from build123d import *

# Parameters (mm, degrees)
SKETCH_1_W                 = 310
SKETCH_1_H                 = 220
EXTRUDE_1_DEPTH            = 12
SKETCH_8_W                 = 310
SKETCH_8_H                 = 10
EXTRUDE_12_DEPTH           = 4
SKETCH_10_R                = 4
CUT_EXTRUDE_5_DEPTH        = 305
SKETCH_11_W                = 4
SKETCH_11_H                = 4
EXTRUDE_13_DEPTH           = 5
EXTRUDE_START              = 300
SKETCH_12_R                = 4
SKETCH_12_R_2              = 3
EXTRUDE_1_2_DEPTH          = 300
SPLIT_START                = -49.339622642
SPLIT_BODIES_2_OUTLINE_R   = 3
SPLIT_BODIES_2_DEPTH       = 100
SPLIT_START_2              = -149.339622642
SPLIT_BODIES_2_2_OUTLINE_R = 3
SPLIT_BODIES_2_2_DEPTH     = 50
SPLIT_START_3              = 100.660377358
SPLIT_BODIES_2_3_OUTLINE_R = 3
SPLIT_BODIES_2_3_DEPTH     = 50
SKETCH_14_W                = 50
SKETCH_14_H                = 8
SKETCH_14_W_2              = 100
EXTRUDE_14_DEPTH           = 12
SKETCH_15_W                = 5
SKETCH_15_H                = 220
EXTRUDE_15_DEPTH           = 5


# Read off the part's stored shape, not the designer's step: 分割2
with BuildPart() as part:
    # 草图1 → Extrude 1 (new body)
    with BuildSketch(Plane(origin=(0, 0, 0), x_dir=(1, 0, 0), z_dir=(0, 1, 0))):
        with Locations((0.660377358, 22.830188679)):
            Rectangle(SKETCH_1_W, SKETCH_1_H)
    extrude(amount=EXTRUDE_1_DEPTH)

    # 草图8 → 凸台-拉伸12 (add)
    with BuildSketch(Plane(origin=(0, 12, 0), x_dir=(1, 0, 0), z_dir=(0, 1, 0))):
        with Locations((0.660377358, 127.830188679)):
            Rectangle(SKETCH_8_W, SKETCH_8_H)
        with Locations((0.660377358, -82.169811321)):
            Rectangle(SKETCH_8_W, SKETCH_8_H)
    extrude(amount=EXTRUDE_12_DEPTH)

    # 草图10 → 切除-拉伸5 (cut)
    with BuildSketch(Plane(origin=(155.660377358, 0, 0), x_dir=(0, 0, -1), z_dir=(1, 0, 0))):
        with Locations((-77.169811321, 16)):
            Circle(SKETCH_10_R)
        with Locations((122.830188679, 16)):
            Circle(SKETCH_10_R)
    extrude(amount=-CUT_EXTRUDE_5_DEPTH, mode=Mode.SUBTRACT)

    # 草图11 → 凸台-拉伸13 (add)
    with BuildSketch(Plane(origin=(155.660377358, 0, 0), x_dir=(0, 0, -1), z_dir=(1, 0, 0))):
        with Locations((-79.169811321, 14)):
            Rectangle(SKETCH_11_W, SKETCH_11_H)
        with Locations((124.830188679, 14)):
            Rectangle(SKETCH_11_W, SKETCH_11_H)
    extrude(amount=-EXTRUDE_13_DEPTH)

    # 草图12 → Extrude 1 2 (add)
    # profile 1 of 2: a face of its own
    with BuildSketch(Plane(origin=(-149.339622642, 0, 0), x_dir=(0, 0, -1), z_dir=(1, 0, 0)).offset(EXTRUDE_START)):
        with Locations((-77.169811321, 16)):
            Circle(SKETCH_12_R)
        with Locations((-77.169811321, 16)):
            Circle(SKETCH_12_R_2, mode=Mode.SUBTRACT)
    # profile 2 of 2: a face of its own
    with BuildSketch(Plane(origin=(-149.339622642, 0, 0), x_dir=(0, 0, -1), z_dir=(1, 0, 0)).offset(EXTRUDE_START)):
        with Locations((122.830188679, 16)):
            Circle(SKETCH_12_R)
        with Locations((122.830188679, 16)):
            Circle(SKETCH_12_R_2, mode=Mode.SUBTRACT)
    extrude(amount=-EXTRUDE_1_2_DEPTH)

    # Split Bodies 2 outline → Split Bodies 2 (cut)
    # profile 1 of 2: a face of its own
    with BuildSketch(Plane.YZ.offset(SPLIT_START)):
        with BuildLine():
            Line((12, -122.830188679), (12, -118.830188679))
            Line((12, -118.830188679), (0, -118.830188679))
            Line((0, -118.830188679), (0, -126.830188679))
            Line((0, -126.830188679), (16, -126.830188679))
            ThreePointArc((16, -126.830188679), (18.828427125, -120.001761554), (12, -122.830188679))
        make_face()
        with Locations((16, -122.830188679)):
            Circle(SPLIT_BODIES_2_OUTLINE_R, mode=Mode.SUBTRACT)
    # profile 2 of 2: a face of its own
    with BuildSketch(Plane.YZ.offset(SPLIT_START)):
        with BuildLine():
            Line((0, 73.169811321), (12, 73.169811321))
            Line((12, 73.169811321), (12, 77.169811321))
            ThreePointArc((12, 77.169811321), (18.828427125, 74.341384196), (16, 81.169811321))
            Line((16, 81.169811321), (0, 81.169811321))
            Line((0, 81.169811321), (0, 73.169811321))
        make_face()
        with Locations((16, 77.169811321)):
            Circle(SPLIT_BODIES_2_OUTLINE_R, mode=Mode.SUBTRACT)
    extrude(amount=SPLIT_BODIES_2_DEPTH, mode=Mode.SUBTRACT)

    # Split Bodies 2 2 outline → Split Bodies 2 2 (cut)
    # profile 1 of 2: a face of its own
    with BuildSketch(Plane.YZ.offset(SPLIT_START_2)):
        with BuildLine():
            Line((12, -122.830188679), (12, -118.830188679))
            Line((12, -118.830188679), (0, -118.830188679))
            Line((0, -118.830188679), (0, -126.830188679))
            Line((0, -126.830188679), (16, -126.830188679))
            ThreePointArc((16, -126.830188679), (18.828427125, -120.001761554), (12, -122.830188679))
        make_face()
        with Locations((16, -122.830188679)):
            Circle(SPLIT_BODIES_2_2_OUTLINE_R, mode=Mode.SUBTRACT)
    # profile 2 of 2: a face of its own
    with BuildSketch(Plane.YZ.offset(SPLIT_START_2)):
        with BuildLine():
            Line((0, 73.169811321), (12, 73.169811321))
            Line((12, 73.169811321), (12, 77.169811321))
            ThreePointArc((12, 77.169811321), (18.828427125, 74.341384196), (16, 81.169811321))
            Line((16, 81.169811321), (0, 81.169811321))
            Line((0, 81.169811321), (0, 73.169811321))
        make_face()
        with Locations((16, 77.169811321)):
            Circle(SPLIT_BODIES_2_2_OUTLINE_R, mode=Mode.SUBTRACT)
    extrude(amount=SPLIT_BODIES_2_2_DEPTH, mode=Mode.SUBTRACT)

    # Split Bodies 2 3 outline → Split Bodies 2 3 (cut)
    # profile 1 of 2: a face of its own
    with BuildSketch(Plane.YZ.offset(SPLIT_START_3)):
        with BuildLine():
            Line((12, -122.830188679), (12, -118.830188679))
            Line((12, -118.830188679), (0, -118.830188679))
            Line((0, -118.830188679), (0, -126.830188679))
            Line((0, -126.830188679), (16, -126.830188679))
            ThreePointArc((16, -126.830188679), (18.828427125, -120.001761554), (12, -122.830188679))
        make_face()
        with Locations((16, -122.830188679)):
            Circle(SPLIT_BODIES_2_3_OUTLINE_R, mode=Mode.SUBTRACT)
    # profile 2 of 2: a face of its own
    with BuildSketch(Plane.YZ.offset(SPLIT_START_3)):
        with BuildLine():
            Line((0, 73.169811321), (12, 73.169811321))
            Line((12, 73.169811321), (12, 77.169811321))
            ThreePointArc((12, 77.169811321), (18.828427125, 74.341384196), (16, 81.169811321))
            Line((16, 81.169811321), (0, 81.169811321))
            Line((0, 81.169811321), (0, 73.169811321))
        make_face()
        with Locations((16, 77.169811321)):
            Circle(SPLIT_BODIES_2_3_OUTLINE_R, mode=Mode.SUBTRACT)
    extrude(amount=SPLIT_BODIES_2_3_DEPTH, mode=Mode.SUBTRACT)

    # 草图14 → 凸台-拉伸14 (add)
    with BuildSketch(Plane(origin=(0, 12, 0), x_dir=(1, 0, 0), z_dir=(0, 1, 0))):
        with Locations((-124.339622642, 122.830188679)):
            Rectangle(SKETCH_14_W, SKETCH_14_H)
        with Locations((125.660377358, 122.830188679)):
            Rectangle(SKETCH_14_W, SKETCH_14_H)
        with Locations((-124.339622642, -77.169811321)):
            Rectangle(SKETCH_14_W, SKETCH_14_H)
        with Locations((125.660377358, -77.169811321)):
            Rectangle(SKETCH_14_W, SKETCH_14_H)
        with Locations((0.660377358, -77.169811321)):
            Rectangle(SKETCH_14_W_2, SKETCH_14_H)
        with Locations((0.660377358, 122.830188679)):
            Rectangle(SKETCH_14_W_2, SKETCH_14_H)
    extrude(amount=-EXTRUDE_14_DEPTH)

    # 草图15 → 凸台-拉伸15 (add)
    with BuildSketch(Plane(origin=(0, 12, 0), x_dir=(1, 0, 0), z_dir=(0, 1, 0))):
        with Locations((-151.839622642, 22.830188679)):
            Rectangle(SKETCH_15_W, SKETCH_15_H)
        with Locations((153.160377358, 22.830188679)):
            Rectangle(SKETCH_15_W, SKETCH_15_H)
    extrude(amount=EXTRUDE_15_DEPTH)


solid = part.part
CAD build for the part. Positions are in the model's coordinates, mm. A direction names the side the tool comes from. Round coordinates to 2 decimals unless told otherwise and drop trailing zeros. Loops run counter-clockwise (first coordinate to the right, second up) from the corner with the lowest first, then second, coordinate; pieces in that order, holes last.
(1) Drop flat-ended pins along their axis: pin 1 (3 mm diameter, centred on x = -63, z = 84, fed in from +Y); pin 2 (12 mm diameter, centred on x = 1.5, z = 53.5, fed in from +Y); pin 3 (5 mm diameter, centred on x = 59.5, z = -128.5, fed in from +Y). Give the stop position or say it passes through.
(2) Cut at B-B (x = -60). Give the cut face in (y, z).
(3) Cut at C-C (x = -10.5). Give the cut face in (y, z), plus the area to 3 significant figures.
(4) Cut at A-A (z = -92.5). Give the cut face in (x, y).
(5) Which spindle directions (+Z, -Z, +X, -X, +Y, -Y) get a long thin tool onto all of the face, cutting with end or side? Do faces 1 (the flat face through (-1, 16, -130)), 2 (the cylindrical face through (76.01, 18.734, 74.25)), 3 (the flat face through (-49.34, 14, 80)), 4 (the flat face through (155.66, 8, -21)). Say none if no direction does.
(6) Wall check: line 1 along Z through (x, y) = (18, 15); line 2 along Z through (x, y) = (-50, 17.5); line 3 along Y through (x, z) = (-54.5, -64.5). Give the ranges that are in metal, low to high.
(7) Two-plate mould, pull along Y, no slides. Class faces 5 (the flat face through (-2, 8, -132.83)), 6 (the cylindrical face through (76.01, 18.92, -120.097)), 7 (the flat face through (-2, 0, -24)): +Y half, -Y half, draft (parallel to the pull), parting line (faces both ways), or undercut.
Findings below:
1. pin 1: stops at y = 16
1. pin 2: stops at y = 12
1. pin 3: stops at y = 18.44
2. outline: (0, -132.83) - (16, -132.83) - (16, -126.83) arc R4 ccw (long way) to (12, -122.83) - (12, 77.17) arc R4 ccw (long way) to (16, 81.17) - (16, 87.17) - (0, 87.17) - close; hole circle Ø6 at (16, -122.83); hole circle Ø6 at (16, 77.17)
3. outline: (0, -132.83) - (16, -132.83) - (16, -126.83) - (12, -126.83) - (12, 81.17) - (16, 81.17) - (16, 87.17) - (0, 87.17) - close
3. area: 2,690 mm2
4. outline: (-154.34, 0) - (155.66, 0) - (155.66, 17) - (150.66, 17) - (150.66, 12) - (-149.34, 12) - (-149.34, 17) - (-154.34, 17) - close
5. face 1: -Z, +Y
5. face 2: none
5. face 3: +Y
5. face 4: +Z, -Z, +X, +Y, -Y
6. line 1: z = -132.83 to -126.83, 81.17 to 87.17
6. line 2: z = -126.54 to -125.43, -120.23 to -119.12, 73.46 to 74.57, 79.77 to 80.88
6. line 3: y = 0 to 12
7. face 5: draft
7. face 6: undercut
7. face 7: -Y half
